Can you work these out from the drawing? Everything is in mm from the part's minimum corner. A direction names the side the tool comes from. Round coordinates to 2 decimals unless told otherwise and drop trailing zeros. Write each loop counter-clockwise with the first axis right and the second up, starting at its lowest first coordinate (ties: lowest second). Pieces come first, ordered by that corner, then holes.
Q1. If we section it at A-A (z = 9.5): Please give me the cut outline in (x, y), plus the area to 3 significant figures.
Q2. I'm going to push flat-ended pins straight in: pin 1 Ø4 at (x, y) = (3.5, 5) entering from +Z; pin 2 Ø4.5 at (y, z) = (25.5, 23.5) entering from -X; pin 3 Ø3 at (y, z) = (22.5, 23.5) entering from +X. Where does each tip first touch, or does it pass through?
Q3. We'd pull the mould along X, two halves only. Please class the marked faces 1, 2, 3 and 4: +X half, -X half, draft (parallel to the pull), parting line (faces both ways), or undercut.
Q4. If we section it at B-B (y = 25): Please give me the cut outline in (x, z).
Q5. If we section it at D-D (z = 2.5): Please give me the cut outline in (x, y), plus the area to 3 significant figures.
Q6. If we section it at C-C (x = 31): Please give me the cut outline in (y, z).
Q7. For the marked faces 5, 6, 7 and 8, which set-ups out of +Z, -Z, +X, -X, +Y, -Y let a thin tool reach every point of the face, with its end or its side?
Q8. Please list where these lines run through material, in increasing order: line 1 along X through (y, z) = (24, 6); line 2 along X through (y, z) = (7.5, 12.5); line 3 along Z through (x, y) = (8, 19.5).
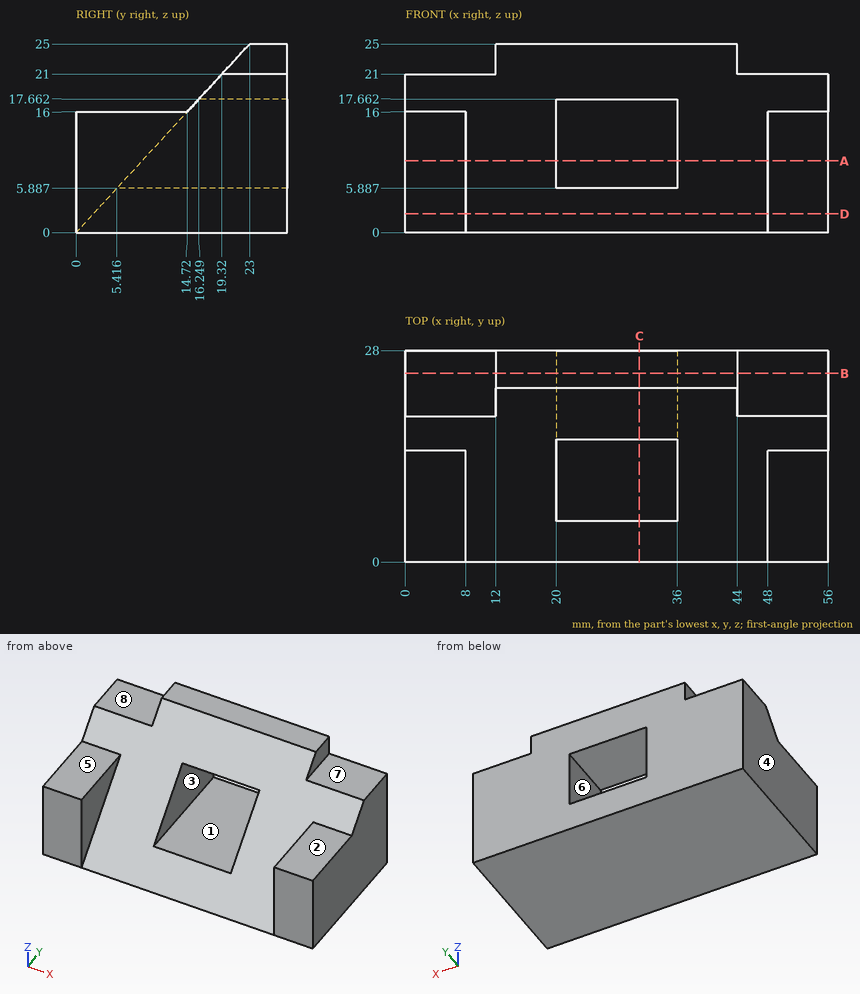
A:
1. outline: (0, 0) - (8, 0) - (8, 8.74) - (20, 8.74) - (20, 28) - (0, 28) - close; (36, 8.74) - (48, 8.74) - (48, 0) - (56, 0) - (56, 28) - (36, 28) - close
1. area: 910 mm2
2. pin 1: stops at z = 16
2. pin 2: stops at x = 12
2. pin 3: stops at x = 44
3. face 1: undercut
3. face 2: draft
3. face 3: undercut
3. face 4: -X half
4. outline: (0, 0) - (56, 0) - (56, 21) - (44, 21) - (44, 25) - (12, 25) - (12, 21) - (0, 21) - close; hole (20, 5.89) - (36, 5.89) - (36, 17.66) - (20, 17.66) - close
5. outline: (0, 0) - (8, 0) - (8, 2.3) - (48, 2.3) - (48, 0) - (56, 0) - (56, 28) - (0, 28) - close
5. area: 1,480 mm2
6. outline: (0, 0) - (28, 0) - (28, 5.89) - (5.42, 5.89) - close; (16.25, 17.66) - (28, 17.66) - (28, 25) - (23, 25) - close
7. face 5: +Z, +X, -X, -Y
7. face 6: +Y, -Y
7. face 7: +Z, +X, +Y, -Y
7. face 8: +Z, -X, +Y, -Y
8. line 1: x = 0 to 20, 36 to 56
8. line 2: x = 0 to 8, 48 to 56
8. line 3: z = 0 to 21
